```python
from build123d import *

# Parameters (mm, degrees)
SKETCH1_R                      = 1.1
MAIN_DEPTH                     = 5
SKETCH2_W                      = 1
SKETCH2_H                      = 2.9
MAKERBEAMSUPPORT_DEPTH         = 26.25
SKETCH3_R                      = 1.6
MAKERBEAMHOLES_DEPTH           = 10
SKETCH4_W                      = 2.6
SKETCH4_H                      = 32.6
CUT_EXTRUDE2_DEPTH             = 12
SKETCH5_W                      = 8
SKETCH5_H                      = 2.9
MAKERBEAMTOPSUPPORT_DEPTH      = 1
SKETCH6_R                      = 1.6
MAKERBEAMTOPHOLESSUPPORT_DEPTH = 12
FILLET1_R                      = 2


with BuildPart() as part:
    # Sketch1 → Main (new body, symmetric)
    with BuildSketch(Plane.XY):
        Polygon((0, 11.3), (-12, 11.3), (-12, 16.3), (-5, 16.3), (-5, 26.3), (3, 26.3), (3, -26.3), (-5, -26.3), (-5, -16.3), (-12, -16.3), (-12, -11.3), (0, -11.3), align=None)
        with Locations((-6, 14)):
            Circle(SKETCH1_R, mode=Mode.SUBTRACT)
        with Locations((-6, -14)):
            Circle(SKETCH1_R, mode=Mode.SUBTRACT)
    extrude(amount=MAIN_DEPTH, both=True)

    # Sketch2 → MakerBeamSupport (add, symmetric)
    with BuildSketch(Plane(origin=(0, 0, 0), x_dir=(1, 0, 0), z_dir=(0, 1, 0))):
        with Locations((3.5, 0)):
            Rectangle(SKETCH2_W, SKETCH2_H)
    extrude(amount=MAKERBEAMSUPPORT_DEPTH, both=True)

    # Sketch3 → MakerBeamHoles (cut, through all)
    with BuildSketch(Plane.ZY.offset(5)):
        with Locations((0, 21.3)):
            Circle(SKETCH3_R)
        with Locations((0, -21.3)):
            Circle(SKETCH3_R)
    extrude(amount=-MAKERBEAMHOLES_DEPTH, mode=Mode.SUBTRACT)

    # Sketch4 → Cut-Extrude2 (cut)
    with BuildSketch(Plane.ZY.offset(12)):
        Rectangle(SKETCH4_W, SKETCH4_H)
    extrude(amount=-CUT_EXTRUDE2_DEPTH, mode=Mode.SUBTRACT)

    # Sketch5 → MakerBeamTopSupport (add)
    with BuildSketch(Plane(origin=(0, 0, 5), x_dir=(-1, 0, 0), z_dir=(0, 0, -1))):
        with Locations((1, 21.3)):
            Rectangle(SKETCH5_W, SKETCH5_H)
        with Locations((1, -21.3)):
            Rectangle(SKETCH5_W, SKETCH5_H)
    extrude(amount=-MAKERBEAMTOPSUPPORT_DEPTH)

    # Sketch6 → MakerBeamTopHolesSupport (cut, through all)
    with BuildSketch(Plane.XY.offset(6)):
        with Locations((-1, 21.3)):
            Circle(SKETCH6_R)
        with Locations((-1, -21.3)):
            Circle(SKETCH6_R)
    extrude(amount=-MAKERBEAMTOPHOLESSUPPORT_DEPTH, mode=Mode.SUBTRACT)

    # Fillet1
    fillet1_edges = [part.edges().sort_by_distance(p)[0] for p in [
        (-5, 16.3, 3.15),
        (-5, -16.3, 3.15),
        (-5, 16.3, -3.15),
        (-5, -16.3, -3.15),
    ]]
    fillet(fillet1_edges, radius=FILLET1_R)


solid = part.part
```
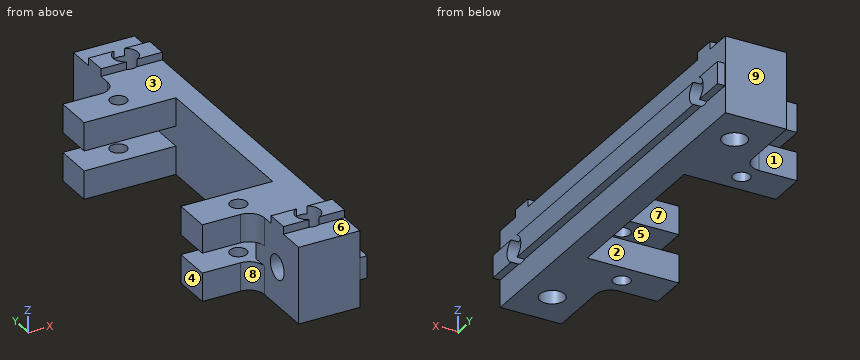
Read the model definition and answer for the solid it produces. Units are mm, in the model's axes. Face numbers are marked on the shaded views. A direction names the side the tool comes from. Coordinates: 2 decimals unless noted, no trailing zeros. Loops run counter-clockwise (first coordinate to the right, second up) from the corner with the lowest first, then second, coordinate; pieces in that order, holes last. Notation, with made-up numbers: (4, 1.5) -> (29, 1.5) arc R21 cw to (29, 13.5) -> close; hole circle Ø2 at (76.25, 18.5). An arc over 180 degrees is marked (long way). Return JSON: item names as keys, results as strings.
Item 1: Find section D-D (y = 14). Determine the outline of the cut face in (x, z), plus the area to 3 significant figures.
Answers:
{"outline": "(-12, -5) -> (-7.1, -5) -> (-7.1, -1.3) -> (-12, -1.3) -> close; (-12, 1.3) -> (-7.1, 1.3) -> (-7.1, 5) -> (-12, 5) -> close; (-4.9, -5) -> (3, -5) -> (3, -1.45) -> (4, -1.45) -> (4, 1.45) -> (3, 1.45) -> (3, 5) -> (-4.9, 5) -> (-4.9, 1.3) -> (0, 1.3) -> (0, -1.3) -> (-4.9, -1.3) -> close", "area": "105 mm2"}
Item 2: Find the intervals of material crossed by probe 1 along Y at (x, z) = (-1, -3.5); probe 2 along X at (y, z) = (14, -3); probe 3 along Z at (x, y) = (-9.5, -14.5), in increasing order.
Answers:
{"probe 1": "y = -26.3 to -22.9, -19.7 to -11.3, 11.3 to 19.7, 22.9 to 26.3", "probe 2": "x = -12 to -7.1, -4.9 to 3", "probe 3": "z = -5 to -1.3, 1.3 to 5"}
Item 3: Find section B-B (y = -21.3). Determine the outline of the cut face in (x, z), plus the area to 3 significant figures.
Answers:
{"outline": "(-5, -5) -> (-2.6, -5) -> (-2.6, -1.6) -> (-5, -1.6) -> close; (-5, 1.6) -> (-2.6, 1.6) -> (-2.6, 6) -> (-5, 6) -> close; (0.6, -5) -> (3, -5) -> (3, -1.6) -> (0.6, -1.6) -> close; (0.6, 1.6) -> (3, 1.6) -> (3, 6) -> (0.6, 6) -> close", "area": "37.4 mm2"}
Item 4: Find section C-C (z = -2.25). Determine the outline of the cut face in (x, y).
Answers:
{"outline": "(-12, -16.3) -> (-7, -16.3) arc R2 cw to (-5, -18.3) -> (-5, -26.3) -> (3, -26.3) -> (3, 26.3) -> (-5, 26.3) -> (-5, 18.3) arc R2 cw to (-7, 16.3) -> (-12, 16.3) -> (-12, 11.3) -> (0, 11.3) -> (0, -11.3) -> (-12, -11.3) -> close; hole circle Ø2.2 at (-6, -14); hole circle Ø2.2 at (-6, 14); hole circle Ø3.2 at (-1, -21.3); hole circle Ø3.2 at (-1, 21.3)"}
Item 5: For the marked faces 1, 2, 3, 4 and 5, determine the directions among +Z, -Z, +X, -X, +Y, -Y from which every point of the face is accessible in a straight line to the end or side of a thin tool.
Answers:
{"face 1": "+Z, -Z, -X, +Y", "face 2": "+Z, -Z, -X", "face 3": "+Z, +X, -X", "face 4": "+Z, -Z, -X, +Y, -Y", "face 5": "-X"}
Item 6: Flat-ended cylindrical pins translate along their axes: P1, Ø0.5, axis at x = 3.5, z = -0.5, coming from the -Y side; P2, Ø3, axis at x = -9, z = 3.5, coming from the +Y side; P3, Ø1.8, axis at x = 0, y = -25.5, coming from the +Z side. Find the tip coordinate at first contact, or state that the pin passes through.
Answers:
{"P1": "stops at y = -26.25", "P2": "stops at y = 16.3", "P3": "stops at z = 5"}
Item 7: Find section A-A (x = -4). Determine the outline of the cut face in (y, z).
Answers:
{"outline": "(-26.3, -5) -> (-11.3, -5) -> (-11.3, -1.3) -> (-16.3, -1.3) -> (-16.3, 1.3) -> (-11.3, 1.3) -> (-11.3, 5) -> (-19.85, 5) -> (-19.85, 6) -> (-22.75, 6) -> (-22.75, 5) -> (-26.3, 5) -> close; (11.3, -5) -> (26.3, -5) -> (26.3, 5) -> (22.75, 5) -> (22.75, 6) -> (19.85, 6) -> (19.85, 5) -> (11.3, 5) -> (11.3, 1.3) -> (16.3, 1.3) -> (16.3, -1.3) -> (11.3, -1.3) -> close; hole circle Ø3.2 at (-21.3, 0); hole circle Ø3.2 at (21.3, 0)"}
Item 8: For a pull along Y with two mould halves and no side action, classify the marked faces 6, 7, 8 and 9 as +Y half, -Y half, draft (parallel to the pull), parting line (faces both ways), or undercut.
Answers:
{"face 6": "draft", "face 7": "undercut", "face 8": "-Y half", "face 9": "+Y half"}
